from build123d import *

# Parameters (mm, degrees)
BOSS_EXTRUDE1_DEPTH             = 4.7752
SKETCH5_R                       = 12.065
CE_00_TUBE_HOLE_DEPTH           = 277.520788418
F_10_32_TAPPED_HOLE1_AT_2_COUNT = 2
F_10_32_TAPPED_HOLE1_AT_2_PITCH = 65.1002
F_10_32_TAPPED_HOLE1_AT_3_COUNT = 2
F_10_32_TAPPED_HOLE1_AT_3_PITCH = 92.075
F_10_32_TAPPED_HOLE1_AT_4_COUNT = 2
F_10_32_TAPPED_HOLE1_AT_4_PITCH = 112.764540814
F_10_32_TAPPED_HOLE1_AT_5_COUNT = 2
F_10_32_TAPPED_HOLE1_AT_5_PITCH = 184.15
F_10_32_TAPPED_HOLE1_AT_6_COUNT = 2
F_10_32_TAPPED_HOLE1_AT_6_PITCH = 195.318351775
F_11_0_191_DIAMETER_HOLE1_D     = 4.8514
F_11_0_191_DIAMETER_HOLE2_D     = 4.8514
CE_00_SHELF_GROOVE_DEPTH        = 1.5748
CE_00_RELIEF_GROOVE_DEPTH       = 2.286
SKETCH18_R                      = 18.2499
SKETCH18_R_2                    = 14.2875
CE_00_TUBE_GASKET_GROOVE_DEPTH  = 3.175
CE_00_TABE_FEATURES_DEPTH       = 277.520788418
FILLET1_R                       = 4.7752
SKETCH22_R                      = 9.525
SKETCH22_R_2                    = 2.0193
CUT_EXTRUDE1_DEPTH              = 277.520788418


with BuildPart() as part:
    # Sketch1 → Boss-Extrude1 (new body)
    with BuildSketch(Plane.XY):
        with BuildLine():
            Line((63.5, 139.7), (139.7, 63.5))
            Line((139.7, 63.5), (139.7, -41.275))
            Line((139.7, -41.275), (-53.975, -234.95))
            Line((-53.975, -234.95), (-56.869763556, -234.95))
            ThreePointArc((-56.869763556, -234.95), (-59.279419133, -235.557868517), (-61.1124, -237.236))
            Line((-61.1124, -237.236), (-65.8876, -237.236))
            ThreePointArc((-65.8876, -237.236), (-67.720580867, -235.557868517), (-70.130236444, -234.95))
            Line((-70.130236444, -234.95), (-139.7, -234.95))
            Line((-139.7, -234.95), (-139.7, -165.380236444))
            ThreePointArc((-139.7, -165.380236444), (-140.307868517, -162.970580867), (-141.986, -161.1376))
            Line((-141.986, -161.1376), (-141.986, -156.3624))
            ThreePointArc((-141.986, -156.3624), (-140.307868517, -154.529419133), (-139.7, -152.119763556))
            Line((-139.7, -152.119763556), (-139.7, 63.5))
            Line((-139.7, 63.5), (-63.5, 139.7))
            Line((-63.5, 139.7), (63.5, 139.7))
        make_face()
    extrude(amount=BOSS_EXTRUDE1_DEPTH)

    # Sketch5 → CE-00 TUbe Hole (cut, through all)
    with BuildSketch(Plane.XY):
        with Locations((117.475, 53.975)):
            Circle(SKETCH5_R)
    extrude(amount=CE_00_TUBE_HOLE_DEPTH, mode=Mode.SUBTRACT)

    # Sketch6 → #10-32 Tapped Hole1 (revolve, cut)
    with BuildSketch(Plane(origin=(-92.075, 95.2754, 0), x_dir=(0, 1, 0), z_dir=(1, 0, 0))):
        Polygon((0, 0), (0, 4.7752), (3.048, 4.7752), (2.0193, 3.7465), (2.0193, 1.0287), (3.048, 0), align=None)
    f_10_32_tapped_hole1 = revolve(axis=Axis((-92.075, 95.2754, -6.35), (0, 0, 1)), mode=Mode.SUBTRACT)

    # #10-32 Tapped Hole1 at 2: #10-32 Tapped Hole1 ×2
    with Locations(*[(0, -i * F_10_32_TAPPED_HOLE1_AT_2_PITCH, 0) for i in range(1, F_10_32_TAPPED_HOLE1_AT_2_COUNT)]):
        add(f_10_32_tapped_hole1, mode=Mode.SUBTRACT)

    # #10-32 Tapped Hole1 at 3: #10-32 Tapped Hole1 ×2
    with Locations(*[(i * F_10_32_TAPPED_HOLE1_AT_3_PITCH, 0, 0) for i in range(1, F_10_32_TAPPED_HOLE1_AT_3_COUNT)]):
        add(f_10_32_tapped_hole1, mode=Mode.SUBTRACT)

    # #10-32 Tapped Hole1 at 4: #10-32 Tapped Hole1 ×2
    with Locations(*[Vector(0.8165244086055451, -0.5773109128982101, 0) * (i * F_10_32_TAPPED_HOLE1_AT_4_PITCH) for i in range(1, F_10_32_TAPPED_HOLE1_AT_4_COUNT)]):
        add(f_10_32_tapped_hole1, mode=Mode.SUBTRACT)

    # #10-32 Tapped Hole1 at 5: #10-32 Tapped Hole1 ×2
    with Locations(*[(i * F_10_32_TAPPED_HOLE1_AT_5_PITCH, 0, 0) for i in range(1, F_10_32_TAPPED_HOLE1_AT_5_COUNT)]):
        add(f_10_32_tapped_hole1, mode=Mode.SUBTRACT)

    # #10-32 Tapped Hole1 at 6: #10-32 Tapped Hole1 ×2
    with Locations(*[Vector(0.9428197520952135, -0.3333030378786251, 0) * (i * F_10_32_TAPPED_HOLE1_AT_6_PITCH) for i in range(1, F_10_32_TAPPED_HOLE1_AT_6_COUNT)]):
        add(f_10_32_tapped_hole1, mode=Mode.SUBTRACT)

    # #11 (0.191) Diameter Hole1 (through all)
    with Locations(Plane(origin=(0, 0, 0), x_dir=(-1, 0, 0), z_dir=(0, 0, -1))):
        with Locations((-22.225, -50.8), (22.225, -50.8)):
            Hole(F_11_0_191_DIAMETER_HOLE1_D / 2)

    # #11 (0.191) Diameter Hole2 (through all)
    with Locations(Plane(origin=(0, 0, 0), x_dir=(-1, 0, 0), z_dir=(0, 0, -1))):
        with Locations((101.6, -19.05), (120.65, -158.75), (63.5, -215.9), (-101.6, -19.05)):
            Hole(F_11_0_191_DIAMETER_HOLE2_D / 2)

    # Sketch20 → #8-32 Tapped Hole1 (revolve, cut)
    with BuildSketch(Plane(origin=(85.725, -50.8, 0), x_dir=(0, 1, 0), z_dir=(1, 0, 0))):
        Polygon((0, 0), (0, 4.7752), (2.286, 4.7752), (1.7272, 4.2164), (1.7272, 0.5588), (2.286, 0), align=None)
    revolve(axis=Axis((85.725, -50.8, -6.35), (0, 0, 1)), mode=Mode.SUBTRACT)

    # Sketch10 → CE-00 Shelf Groove (cut)
    with BuildSketch(Plane.XY):
        with BuildLine():
            Line((-162.687, 8.763), (158.242, 8.763))
            Line((158.242, 8.763), (158.242, -51.188217219))
            Line((158.242, -51.188217219), (139.954, -51.188217219))
            Line((139.954, -51.188217219), (139.954, 3.175))
            ThreePointArc((139.954, 3.175), (139.02406403, 5.42006403), (136.779, 6.35))
            Line((136.779, 6.35), (-134.112, 6.35))
            ThreePointArc((-134.112, 6.35), (-136.35706403, 5.42006403), (-137.287, 3.175))
            Line((-137.287, 3.175), (-137.287, -15.875))
            ThreePointArc((-137.287, -15.875), (-139.370056572, -20.903943428), (-144.399, -22.987))
            Line((-144.399, -22.987), (-162.687, -22.987))
            Line((-162.687, -22.987), (-162.687, 8.763))
        make_face()
    extrude(amount=CE_00_SHELF_GROOVE_DEPTH, mode=Mode.SUBTRACT)

    # Sketch17 → CE-00 Relief Groove (cut)
    with BuildSketch(Plane(origin=(0, 0, 0), x_dir=(-1, 0, 0), z_dir=(0, 0, -1))):
        with BuildLine():
            Line((130.9624, -2.667), (-133.604, -2.667))
            ThreePointArc((-133.604, -2.667), (-136.906, 0.635), (-133.604, 3.937))
            Line((-133.604, 3.937), (130.9624, 3.937))
            ThreePointArc((130.9624, 3.937), (134.2644, 0.635), (130.9624, -2.667))
        make_face()
    extrude(amount=-CE_00_RELIEF_GROOVE_DEPTH, mode=Mode.SUBTRACT)

    # Sketch18 → CE-00 Tube Gasket Groove (cut)
    with BuildSketch(Plane(origin=(0, 0, 0), x_dir=(-1, 0, 0), z_dir=(0, 0, -1))):
        with Locations((-117.475, 53.721)):
            Circle(SKETCH18_R)
        with Locations((-117.475, 53.721)):
            Circle(SKETCH18_R_2, mode=Mode.SUBTRACT)
    extrude(amount=-CE_00_TUBE_GASKET_GROOVE_DEPTH, mode=Mode.SUBTRACT)

    # Sketch19 → CE-00 Tabe Features (cut, through all)
    with BuildSketch(Plane.XY):
        with BuildLine():
            Line((-141.986, -156.3624), (-141.986, -161.1376))
            Line((-141.986, -161.1376), (-140.462, -161.1376))
            ThreePointArc((-140.462, -161.1376), (-137.922, -163.6776), (-140.462, -166.2176))
            Line((-140.462, -166.2176), (-144.526, -166.2176))
            Line((-144.526, -166.2176), (-144.526, -151.2824))
            Line((-144.526, -151.2824), (-140.462, -151.2824))
            ThreePointArc((-140.462, -151.2824), (-137.922, -153.8224), (-140.462, -156.3624))
            Line((-140.462, -156.3624), (-141.986, -156.3624))
        make_face()
        with BuildLine():
            Line((-61.1124, -237.236), (-65.8876, -237.236))
            Line((-65.8876, -237.236), (-65.8876, -235.712))
            ThreePointArc((-65.8876, -235.712), (-68.4276, -233.172), (-70.9676, -235.712))
            Line((-70.9676, -235.712), (-70.9676, -244.467339737))
            Line((-70.9676, -244.467339737), (-56.0324, -244.467339737))
            Line((-56.0324, -244.467339737), (-56.0324, -235.712))
            ThreePointArc((-56.0324, -235.712), (-58.5724, -233.172), (-61.1124, -235.712))
            Line((-61.1124, -235.712), (-61.1124, -237.236))
        make_face()
    extrude(amount=CE_00_TABE_FEATURES_DEPTH, mode=Mode.SUBTRACT)

    # Fillet1
    fillet1_edges = [part.edges().sort_by_distance(p)[0] for p in [
        (-139.7, -234.95, 2.3876),
        (-139.7, 63.5, 2.3876),
        (-63.5, 139.7, 2.3876),
        (63.5, 139.7, 2.3876),
        (139.7, 63.5, 2.3876),
        (139.7, -41.275, 2.3876),
    ]]
    fillet(fillet1_edges, radius=FILLET1_R)

    # Sketch22 → Cut-Extrude1 (cut, through all)
    with BuildSketch(Plane.XY):
        with Locations((-107.95, -19.05)):
            Circle(SKETCH22_R)
        with Locations((-88.900016933, -19.0754)):
            Circle(SKETCH22_R_2)
    extrude(amount=CUT_EXTRUDE1_DEPTH, mode=Mode.SUBTRACT)


solid = part.part
Verification items for the finished model (mm, model axes). A direction names the side the tool comes from. Coordinates: 2 decimals unless noted, no trailing zeros. Order: outer loops, then holes, each group sorted by start corner. A loop starts at its lowest first (then second) coordinate and runs counter-clockwise, first axis right, second up. Notation, with made-up numbers: M 66,48.25 L 102,48.25 A4 ccw 102,53.25 Z; hole C -4,50.25 d6. An arc over 180 degrees is marked long. One line per item, written item: value. Start each with the question number.
Item 1: Access from +Z, -Z, +X, -X, +Y, -Y to the whole of each face (thin tool, end or side, straight path). Record for faces 1 (the cylindrical face through (128.813, 45.027, 1.565)), 2 (the cylindrical face through (-117.466, -18.631, 2.354)).
Item 2: Depth check by flat-ended pin: P1, Ø1.2, axis at x = -141.5, z = 1.5, coming from the +Y side; P2, Ø0.8, axis at y = -236.5, z = 3.5, coming from the -X side; P3, Ø0.7, axis at x = 7, z = 1.5, coming from the -Y side (3 decimals); P4, Ø17, axis at x = -107.95, y = -19.05, coming from the +Z side. Enter the tip coordinate at first touch or a pass-through.
Item 3: Mould release check, pull along Y, two halves, no side actions. Record for faces 3 (the flat face through (-30, -46, 4.775)), 4 (the flat face through (109, 42, 3.175)), 5 (the flat face through (101.1, 102.1, 2.4)): pulls with the +Y half, pulls with the -Y half, needs draft (parallel to the pull), parting line crosses it, or undercut.
Item 4: Sectioned sample at B-B on y = 79. Record the cut outline in (x, z), then the cut area to 3 significant figures.
Item 5: Sectioned sample at C-C on x = -30. Record the cut outline in (y, z) (3 decimals).
Item 6: Sectioned sample at A-A on x = -107.95. Record the cut outline in (y, z) (3 decimals), then the cut area to 3 significant figures.
Item 7: Thickness scan on probe 1 along Y at (x, z) = (-38, 0.95) (3 decimals); probe 2 along Y at (x, z) = (79.5, 0.95) (3 decimals); probe 3 along Y at (x, z) = (-105.5, 0.3). Record the ranges inside material, lowest first.
Calculated:
1. face 1: -Z
1. face 2: +Z, -Z
2. P1: y = -156.36
2. P2: x = -65.89
2. P3: y = -174.325
2. P4: through
3. face 3: needs draft
3. face 4: undercut
3. face 5: pulls with the +Y half
4. outline: M -124.2,0 L 124.2,0 L 124.2,4.78 L -124.2,4.78 Z
4. area: 1,190 mm^2
5. outline: M -210.975,0 L -2.667,0 L -2.667,2.286 L 3.937,2.286 L 3.937,0 L 6.35,0 L 6.35,1.575 L 8.763,1.575 L 8.763,0 L 139.7,0 L 139.7,4.775 L -210.975,4.775 Z
6. outline: M -234.95,0 L -28.575,0 L -28.575,4.775 L -234.95,4.775 Z; M -9.525,0 L -2.667,0 L -2.667,2.286 L 3.937,2.286 L 3.937,0 L 6.35,0 L 6.35,1.575 L 8.763,1.575 L 8.763,0 L 95.25,0 L 95.25,4.775 L -9.525,4.775 Z
6. area: 1,470 mm^2
7. probe 1: -218.975 to -2.667, 3.937 to 6.35, 8.763 to 139.7
7. probe 2: -101.475 to -2.667, 3.937 to 6.35, 8.763 to 123.7
7. probe 3: -234.95 to -28.25, -9.85 to -2.67, 3.94 to 6.35, 8.76 to 97.7
